from build123d import *

# Parameters (mm, degrees)
F1_DEPTH = 12.7
F0_R     = 3.9116
F2_DEPTH = 6.35
F3_DEPTH = 6.35


# Not quite as in the source:
# - a length typed as a fraction of an inch, garbled in the dataset ("3 / 203.2 mm" for 3/8 in), is restored


with BuildPart() as f1:
    # F0 (on Right) → F1 (new body)
    with BuildSketch(Plane.YZ):
        Polygon((16.66875, -5.55625), (16.66875, 5.55625), (16.66875, 16.66875), (-16.66875, 16.66875), (-16.66875, 5.55625), (-16.66875, -5.55625), (-16.66875, -5.56895), (-16.66875, -16.66875), (16.66875, -16.66875), (16.66875, -5.56895), align=None)
        Polygon((-4.4120975668, 5.55625), (-3.81, 6.5991135768), (3.81, 6.5991135768), (4.4120975668, 5.55625), (7.62, 0), (4.4120975668, -5.55625), (3.81, -6.5991135768), (-3.81, -6.5991135768), (-4.4120975668, -5.55625), (-7.62, 0), align=None, mode=Mode.SUBTRACT)
        Polygon((-16.66875, -5.55625), (-16.66875, 5.55625), (-46.84395, 5.55625), (-46.84395, -5.56895), (-16.66875, -5.56895), align=None)
        Polygon((46.83125, 5.55625), (16.66875, 5.55625), (16.66875, -5.55625), (16.66875, -5.56895), (46.83125, -5.56895), align=None)
    extrude(amount=F1_DEPTH)

    # F0 (on Right) → F2 (join)
    with BuildSketch(Plane.YZ):
        Polygon((3.81, 6.5991135768), (-3.81, 6.5991135768), (-4.4120975668, 5.55625), (-7.62, 0), (-4.4120975668, -5.55625), (-3.81, -6.5991135768), (3.81, -6.5991135768), (4.4120975668, -5.55625), (7.62, 0), (4.4120975668, 5.55625), align=None)
        Circle(F0_R, mode=Mode.SUBTRACT)
    extrude(amount=F2_DEPTH)

    # F0 (on Right) → F3 (cut)
    with BuildSketch(Plane.YZ):
        Polygon((-16.66875, -5.55625), (-16.66875, 5.55625), (-46.84395, 5.55625), (-46.84395, -5.56895), (-16.66875, -5.56895), align=None)
        Polygon((46.83125, 5.55625), (16.66875, 5.55625), (16.66875, -5.55625), (16.66875, -5.56895), (46.83125, -5.56895), align=None)
    extrude(amount=F3_DEPTH, mode=Mode.SUBTRACT)


solid = f1.part
Model file for the job. Use its own axes, mm. A direction names the side the tool comes from. Give positions to 0.01 mm unless a question says otherwise; leave off trailing zeros. Loops run counter-clockwise (first coordinate to the right, second up) from the corner with the lowest first, then second, coordinate; pieces in that order, holes last. Notation, with made-up numbers: (19.5, 0.5) - (25.5, 0.5) arc R8 ccw to (25.5, 6.5) - close; hole circle Ø10 at (7, 14.5). An arc over 180 degrees is marked (long way). Use one line per item in the form item = value.
(1) Drill centre lines: L1, parallel to Z at x = 2.5, y = 0; L2, parallel to Z at x = 6.75, y = 3.5; L3, parallel to Y at x = 1.25, z = -8. Where is each one in solid material? Low to high.
Determined:
L1 = -16.67 to -3.91, 3.91 to 16.67
L2 = -16.67 to -6.6, 6.6 to 16.67
L3 = -16.67 to 16.67
(2) Cut at D-D (x = 2.75). Give the cut face in (y, z).
Determined:
outline = (-16.67, -16.67) - (16.67, -16.67) - (16.67, 16.67) - (-16.67, 16.67) - close; hole circle Ø7.82 at (0, 0)
(3) Cut at A-A (y = 0). Give the cut face in (x, z).
Determined:
outline = (0, -16.67) - (12.7, -16.67) - (12.7, -6.6) - (6.35, -6.6) - (6.35, -3.91) - (0, -3.91) - close; (0, 3.91) - (6.35, 3.91) - (6.35, 6.6) - (12.7, 6.6) - (12.7, 16.67) - (0, 16.67) - close
(4) Cut at B-B (x = 10.25). Give the cut face in (y, z).
Determined:
outline = (-46.84, -5.57) - (-16.67, -5.57) - (-16.67, -16.67) - (16.67, -16.67) - (16.67, -5.57) - (46.83, -5.57) - (46.83, 5.56) - (16.67, 5.56) - (16.67, 16.67) - (-16.67, 16.67) - (-16.67, 5.56) - (-46.84, 5.56) - close; hole (-7.62, 0) - (-3.81, -6.6) - (3.81, -6.6) - (7.62, 0) - (3.81, 6.6) - (-3.81, 6.6) - close
(5) 3-axis set-ups, long thin cutter, end or side, ignore diameter. For faces 1 (the face through (9, -32, -5.569)), 2 (the face through (9, -32, 5.556)), 3 (the face through (6.35, -32, 0)), 4 (the face through (9, 0, -6.599)): which of +Z, -Z, +X, -X, +Y, -Y reach the whole face in a straight line?
Determined:
face_1 = -Z, +X, -X, -Y
face_2 = +Z, +X, -X, -Y
face_3 = +Z, -Z, -X, -Y
face_4 = +X
(6) Drop flat-ended pins along their axis: P1, Ø5, axis at x = 8.5, y = 33.5, coming from the +Z side; P2, Ø2, axis at x = 5, z = -2.5, coming from the -Y side; P3, Ø5, axis at x = 10, y = 37.5, coming from the -Z side. Give the stop position or say it passes through.
Determined:
P1 = 5.56
P2 = -16.67
P3 = -5.57
(7) Pull direction Z, two halves, no side cores. Call faces 5 (the face through (6.35, 32, 0)), 6 (the face through (9, 32, 5.556)), 7 (the face through (9, 0, 6.599)): pulls with the +Z half, pulls with the -Z half, needs draft (parallel to the pull), parting line crosses it, or undercut.
Determined:
face_5 = needs draft
face_6 = pulls with the +Z half
face_7 = undercut
(8) Cut at C-C (z = 10). Give the cut face in (x, y), then the cut area to 3 significant figures.
Determined:
outline = (0, -16.67) - (12.7, -16.67) - (12.7, 16.67) - (0, 16.67) - close
area = 423 mm^2
